CAD build for the part. Positions are in the model's coordinates, mm. A direction names the side the tool comes from. Give positions to 0.01 mm unless a question says otherwise; leave off trailing zeros. Write each loop counter-clockwise with the first axis right and the second up, starting at its lowest first coordinate (ties: lowest second). Pieces come first, ordered by that corner, then holes. Notation, with made-up numbers: (86, 58) -> (135, 58) arc R22 cw to (135, 80) -> close; hole circle Ø6 at (24.5, 51.5). An arc over 180 degrees is marked (long way). Use one line per item in the form item = value. Start each with the question number.
from build123d import *

# Parameters (mm, degrees)
BOSS_EXTRUDE1_DEPTH         = 6.35
TAP_DRILL_FOR_8_HELICOIL2_D = 4.3942
SKETCH5_R                   = 14.2875
CUT_EXTRUDE1_DEPTH          = 3.175
SKETCH6_W                   = 13.215231571
SKETCH6_H                   = 25.4
SKETCH6_W_2                 = 16.390231571
SKETCH6_H_2                 = 28.575
CUT_EXTRUDE2_DEPTH          = 3.175
FILLET1_R                   = 7.62
SKETCH7_R                   = 8.255
CUT_EXTRUDE3_DEPTH          = 47.513779973


with BuildPart() as part:
    # Sketch2 → Boss-Extrude1 (new body)
    with BuildSketch(Plane.XY):
        with BuildLine():
            Line((0, 0), (-19.05, -9.525))
            ThreePointArc((-19.05, -9.525), (-25.915231571, -19.05), (-19.05, -28.575))
            Line((-19.05, -28.575), (0, -38.1))
            Line((0, -38.1), (19.05, -28.575))
            ThreePointArc((19.05, -28.575), (25.915231571, -19.05), (19.05, -9.525))
            Line((19.05, -9.525), (0, 0))
        make_face()
    extrude(amount=BOSS_EXTRUDE1_DEPTH)

    # Tap Drill for #8 Helicoil2 (through all)
    with Locations(Plane.XY.offset(6.35)):
        with Locations((-19.05, -19.05), (19.05, -19.05)):
            Hole(TAP_DRILL_FOR_8_HELICOIL2_D / 2)

    # Sketch5 → Cut-Extrude1 (cut)
    with BuildSketch(Plane.XY.offset(6.35)):
        with Locations((0, -19.05)):
            Circle(SKETCH5_R)
    extrude(amount=-CUT_EXTRUDE1_DEPTH, mode=Mode.SUBTRACT)

    # Sketch6 → Cut-Extrude2 (cut)
    with BuildSketch(Plane(origin=(0, 0, 0), x_dir=(-1, 0, 0), z_dir=(0, 0, -1))):
        with Locations((19.307615786, -19.05)):
            Rectangle(SKETCH6_W, SKETCH6_H)
        with Locations((-17.720115786, -19.05)):
            Rectangle(SKETCH6_W_2, SKETCH6_H_2)
    extrude(amount=-CUT_EXTRUDE2_DEPTH, mode=Mode.SUBTRACT)

    # Fillet1
    # the kernel refuses this fillet: 7.62 mm, written as the material it takes off along each edge
    with BuildSketch(Plane(origin=(-12.7, -31.75, -11.773547486), x_dir=(0.8944271909999157, -0.44721359549995826, 0), z_dir=(0, 0, 1)), Plane(origin=(-12.7, -6.35, -11.773547486), x_dir=(0, -1, 0), z_dir=(0, 0, 1)), Plane(origin=(9.525, -4.7625, -11.773547486), x_dir=(-0.894427190999916, 0.4472135954999576, 0), z_dir=(0, 0, 1))) as fillet1_piece_1:
        with BuildLine():
            CenterArc((FILLET1_R * 0.61803398875, FILLET1_R), FILLET1_R, 206.565051177, 63.434948823)
            Line((-FILLET1_R * 0.27639320225, FILLET1_R * 0.5527864045), (0, 0))
            Line((0, 0), (FILLET1_R * 0.61803398875, 0))
        make_face()
    extrude(amount=14.948547486, mode=Mode.SUBTRACT)
    with BuildSketch(Plane(origin=(9.525, -33.3375, -11.773547486), x_dir=(-0.8944271909999163, -0.4472135954999572, 0), z_dir=(0, 0, 1))) as fillet1_piece_2:
        with BuildLine():
            CenterArc((FILLET1_R * 0.61803398875, -FILLET1_R), FILLET1_R, 90, 63.434948823)
            Line((-FILLET1_R * 0.27639320225, -FILLET1_R * 0.5527864045), (0, 0))
            Line((0, 0), (FILLET1_R * 0.61803398875, 0))
        make_face()
    extrude(amount=14.948547486, mode=Mode.SUBTRACT)

    # Sketch7 → Cut-Extrude3 (cut, through all)
    with BuildSketch(Plane(origin=(0, 0, 0), x_dir=(-1, 0, 0), z_dir=(0, 0, -1))):
        with Locations((0, -19.05)):
            Circle(SKETCH7_R)
    extrude(amount=-CUT_EXTRUDE3_DEPTH, mode=Mode.SUBTRACT)


solid = part.part
1) 3-axis set-ups, long thin cutter, end or side, ignore diameter. For faces 4 (the face through (-11.59, -31, 1.57)), 5 (the face through (-11.53, -7, 1.57)), 6 (the face through (-7.874, -16.57, 1.565)), 7 (the face through (8.42, -5.52, 1.57)), 8 (the face through (-9, -19, 3.175)): which of +Z, -Z, +X, -X, +Y, -Y reach the whole face in a straight line?
2) Cut at A-A (z = 4.5). State how many separate pieces and enclosed holes the cut face has, and give its area (3 significant figures).
3) Wall check: line 1 along Y through (x, z) = (0, 2.45) (3 decimals); line 2 along Z through (x, y) = (15.5, -15) (3 decimals); line 3 along Y through (x, z) = (-19.05, 4.35) (3 decimals). Give the ranges that are in metal, low to high. Write a range as from..to.
4) Two-plate mould, pull along X, no slides. Class faces 1 (the face through (8.36, -32.68, 1.57)), 2 (the face through (-15, -19, 3.175)), 3 (the face through (-3.097, -32.998, 4.785)): released by +X, released by -X, zero draft, split by the parting line, or undercut.
5) Pin check, flat tips, straight feed: pin 1 (6 mm diameter, centred on x = -19, y = -13, fed in from -Z) (3 decimals); pin 2 (1.5 mm diameter, centred on x = -12.5, z = 1.5, fed in from -Y); pin 3 (3.5 mm diameter, centred on y = -19.5, z = 1, fed in from -X); pin 4 (3 mm diameter, centred on x = -15.5, y = -34, fed in from +Z). Stop position of each tip, or through.
6) Cut at C-C (x = 20). Give the cut face in (y, z) (3 decimals), and give its area (3 significant figures).
7) Cut at D-D (y = -31.5). Give the cut face in (x, z) (3 decimals).
Final values:
q1.face_4 = -Z, -X, -Y
q1.face_5 = -Z, -X, +Y
q1.face_6 = +Z, -Z
q1.face_7 = -Z, +X, +Y
q1.face_8 = +Z
q2.separate_pieces = 1
q2.enclosed_holes = 3
q2.area = 608 mm^2
q3.line_1 = -38.1..-27.305, -10.795..0
q3.line_2 = 3.175..6.35
q3.line_3 = -28.575..-21.247, -16.853..-9.525
q4.face_1 = released by +X
q4.face_2 = zero draft
q4.face_3 = undercut
q5.pin_1 = 3.175
q5.pin_2 = -30.73
q5.pin_3 = -12.7
q5.pin_4 = through
q6.outline = (-28.204, 3.175) -> (-21.031, 3.175) -> (-21.031, 6.35) -> (-28.204, 6.35) -> close; (-17.069, 3.175) -> (-9.896, 3.175) -> (-9.896, 6.35) -> (-17.069, 6.35) -> close
q6.area = 45.5 mm^2
q7.outline = (-13.2, 3.175) -> (-11.259, 3.175) -> (-11.259, 0) -> (8.963, 0) -> (8.963, 3.175) -> (13.2, 3.175) -> (13.2, 6.35) -> (7.009, 6.35) -> (7.009, 3.175) -> (-7.009, 3.175) -> (-7.009, 6.35) -> (-13.2, 6.35) -> close
